Build history of the part. All positions in model axes, mm. Face numbers are marked on the shaded views. A direction names the side the tool comes from. Round coordinates to 2 decimals unless told otherwise and drop trailing zeros. Write each loop counter-clockwise with the first axis right and the second up, starting at its lowest first coordinate (ties: lowest second). Pieces come first, ordered by that corner, then holes. Notation, with made-up numbers: (60, -1.5) -> (87, -1.5) arc R15 cw to (87, 14.5) -> close; hole circle Ø4 at (-26.75, 56). An arc over 180 degrees is marked (long way). Answer in a Markdown table with one row per item.
```python
from build123d import *

# Parameters (mm, degrees)
F0_W      = 4.1414871812
F0_H      = 2.5
F0_W_2    = 6.3956826925
F0_W_3    = 4.0508699417
F0_W_4    = 5.4119601846
F0_W_5    = 25
F0_H_2    = 35.3582080007
F0_R      = 3.9974062239
F0_W_6    = 20
F0_H_3    = 12.5
F1_DEPTH  = 3
F2_DEPTH  = 5
F3_DEPTH  = 1.4
F0_R_2    = 3
F4_DEPTH  = 5
F5_DEPTH  = 3
F7_DEPTH  = 5
F9_DEPTH  = 5
F10_R     = 3
F11_DEPTH = 2


with BuildPart() as f1:
    # F0 (on Top) → F1 (new body)
    with BuildSketch(Plane.XY):
        with Locations((-2.0707435906, -1.25)):
            Rectangle(F0_W, F0_H)
        with Locations((-7.3393285275, -1.25)):
            Rectangle(F0_W_2, F0_H)
        with Locations((-17.9745650291, -1.25)):
            Rectangle(F0_W_3, F0_H)
        with Locations((-13.243149966, -1.25)):
            Rectangle(F0_W_4, F0_H)
        Polygon((0, 12), (0, 0), (0, -2.5), (2.5, -2.5), (2.5, 27), (-22.5, 27), (-22.5, -2.5), (-20, -2.5), (-20, 0), (-20, 12), (-20, 24.5), (0, 24.5), align=None)
        with Locations((-10, 44.6791040003)):
            Rectangle(F0_W_5, F0_H_2)
        with Locations((-10, 54.3582080007)):
            Circle(F0_R, mode=Mode.SUBTRACT)
        with Locations((-10, 18.25)):
            Rectangle(F0_W_6, F0_H_3)
        Polygon((-4.1414871812, 0), (0, 0), (0, 12), (-20, 12), (-20, 0), (-15.9491300583, 0), (-10.5371698737, 0), align=None)
    extrude(amount=-F1_DEPTH)

    # F0 (on Top) → F2 (join)
    with BuildSketch(Plane.XY):
        Polygon((0, 12), (0, 0), (0, -2.5), (2.5, -2.5), (2.5, 27), (-22.5, 27), (-22.5, -2.5), (-20, -2.5), (-20, 0), (-20, 12), (-20, 24.5), (0, 24.5), align=None)
        with Locations((-7.3393285275, -1.25)):
            Rectangle(F0_W_2, F0_H)
    extrude(amount=F2_DEPTH)

    # F0 (on Top) → F3 (join)
    with BuildSketch(Plane.XY):
        with Locations((-10, 18.25)):
            Rectangle(F0_W_6, F0_H_3)
    extrude(amount=F3_DEPTH)

    # F0 (on Top) → F4 (join)
    with BuildSketch(Plane.XY):
        with Locations((-10, 54.3582080007)):
            Circle(F0_R)
        with Locations((-10, 54.3582080007)):
            Circle(F0_R_2, mode=Mode.SUBTRACT)
    extrude(amount=F4_DEPTH)

    # F0 (on Top) → F5 (join)
    with BuildSketch(Plane.XY):
        with Locations((-10, 54.3582080007)):
            Circle(F0_R)
        with Locations((-10, 54.3582080007)):
            Circle(F0_R_2, mode=Mode.SUBTRACT)
        with Locations((-10, 54.3582080007)):
            Circle(F0_R_2)
    extrude(amount=-F5_DEPTH)

    # F6 (on face) → F7 (join)
    with BuildSketch(Plane.YZ.offset(2.5)):
        with BuildLine():
            ThreePointArc((41, 7), (38, 10), (35, 7))
            Line((35, 7), (36.25, 7))
            ThreePointArc((36.25, 7), (38, 8.75), (39.75, 7))
            Line((39.75, 7), (41, 7))
        make_face()
        with BuildLine():
            Line((35, 7), (35, 0))
            Line((35, 0), (41, 0))
            Line((41, 0), (41, 7))
            Line((41, 7), (39.75, 7))
            ThreePointArc((39.75, 7), (38, 5.25), (36.25, 7))
            Line((36.25, 7), (35, 7))
        make_face()
    extrude(amount=-F7_DEPTH)

    # F8 (on face) → F9 (join)
    with BuildSketch(Plane(origin=(-22.5, 0, 0), x_dir=(0, -1, 0), z_dir=(-1, 0, 0))):
        with BuildLine():
            Line((-41, 7), (-41, 0))
            Line((-41, 0), (-35, 0))
            Line((-35, 0), (-35, 7))
            Line((-35, 7), (-36.25, 7))
            ThreePointArc((-36.25, 7), (-38, 5.25), (-39.75, 7))
            Line((-39.75, 7), (-41, 7))
        make_face()
        with BuildLine():
            ThreePointArc((-35, 7), (-38, 10), (-41, 7))
            Line((-41, 7), (-39.75, 7))
            ThreePointArc((-39.75, 7), (-38, 8.75), (-36.25, 7))
            Line((-36.25, 7), (-35, 7))
        make_face()
    extrude(amount=-F9_DEPTH)

    # F10 (on face) → F11 (join)
    with BuildSketch(Plane(origin=(0, 0, -3), x_dir=(1, 0, 0), z_dir=(0, 0, -1))):
        with Locations((-10, -54.3582080007)):
            Circle(F10_R)
    extrude(amount=-F11_DEPTH)


solid = f1.part
```
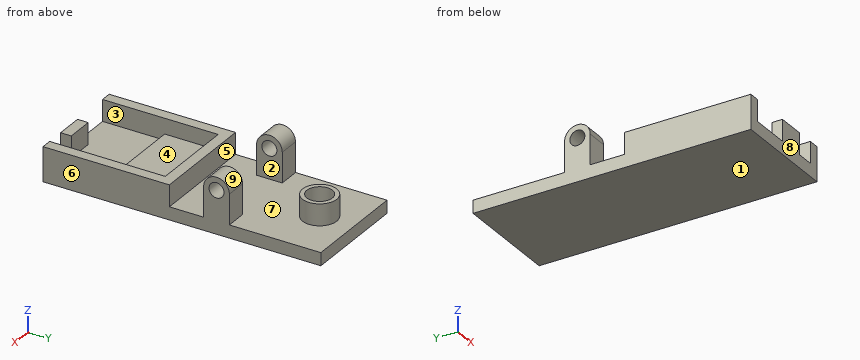
Q1. Saw through at D-D on y = 29. Write the cut outline in (x, z), plus the area to 3 significant figures.
A:
| item | result |
|---|---|
| outline | (-22.5, -3) -> (2.5, -3) -> (2.5, 0) -> (-22.5, 0) -> close |
| area | 75.0 mm² |
Q2. Drop flat-ended pins along their axis: P1, Ø1.2, axis at x = -8.5, y = -1.5, coming from the +Z side; P2, Ø1, axis at x = -12.5, z = 4, coming from the -Y side; P3, Ø2.5, axis at x = -10, z = 2, coming from the +Y side. Give the stop position or say it passes through.
A:
| item | result |
|---|---|
| P1 | z = 5 |
| P2 | y = 24.5 |
| P3 | y = 58.36 |
Q3. Saw through at A-A on z = 3. Write the cut outline in (x, y), plus the area to 3 significant figures.
A:
| item | result |
|---|---|
| outline | (-22.5, -2.5) -> (-20, -2.5) -> (-20, 24.5) -> (0, 24.5) -> (0, -2.5) -> (2.5, -2.5) -> (2.5, 27) -> (-22.5, 27) -> close; (-22.5, 35) -> (-17.5, 35) -> (-17.5, 41) -> (-22.5, 41) -> close; circle Ø7.99 at (-10, 54.36); (-10.54, -2.5) -> (-4.14, -2.5) -> (-4.14, 0) -> (-10.54, 0) -> close; (-2.5, 35) -> (2.5, 35) -> (2.5, 41) -> (-2.5, 41) -> close; hole circle Ø6 at (-10, 54.36) |
| area | 295 mm² |
Q4. Saw through at B-B on y = 38. Write the cut outline in (x, z).
A:
| item | result |
|---|---|
| outline | (-22.5, -3) -> (2.5, -3) -> (2.5, 5.25) -> (-2.5, 5.25) -> (-2.5, 0) -> (-17.5, 0) -> (-17.5, 5.25) -> (-22.5, 5.25) -> close; (-22.5, 8.75) -> (-17.5, 8.75) -> (-17.5, 10) -> (-22.5, 10) -> close; (-2.5, 8.75) -> (2.5, 8.75) -> (2.5, 10) -> (-2.5, 10) -> close |
Q5. Saw through at C-C on y = 17.5. Write the cut outline in (x, z), plus the area to 3 significant figures.
A:
| item | result |
|---|---|
| outline | (-22.5, -3) -> (2.5, -3) -> (2.5, 5) -> (0, 5) -> (0, 1.4) -> (-20, 1.4) -> (-20, 5) -> (-22.5, 5) -> close |
| area | 128 mm² |
Q6. Which spindle directions (+Z, -Z, +X, -X, +Y, -Y) get a long thin tool onto all of the face, cutting with end or side? Do the marked faces 1, 2, 3, 4 and 5. Say none if no direction does.
A:
| item | result |
|---|---|
| face 1 | -Z, +X, -X, +Y, -Y |
| face 2 | +Z, +Y |
| face 3 | +Z, -Y |
| face 4 | +Z |
| face 5 | +Z, +X, -X |
Q7. Wall check: line 1 (Y direction, x = 1, z = 7); line 2 (X direction, y = 38.5, z = 0.75); line 3 (Z direction, x = -20.7, y = 38). Give the ranges that are in metal, low to high. Write a range as [from, to].
A:
| item | result |
|---|---|
| line 1 | [35, 36.25], [39.75, 41] |
| line 2 | [-22.5, -17.5], [-2.5, 2.5] |
| line 3 | [-3, 5.25], [8.75, 10] |
Q8. Two-plate mould, pull along Y, no slides. Class the marked faces 6, 7, 8 and 9: released by +Y, released by -Y, zero draft, split by the parting line, or undercut.
A:
| item | result |
|---|---|
| face 6 | zero draft |
| face 7 | undercut |
| face 8 | released by -Y |
| face 9 | split by the parting line |
